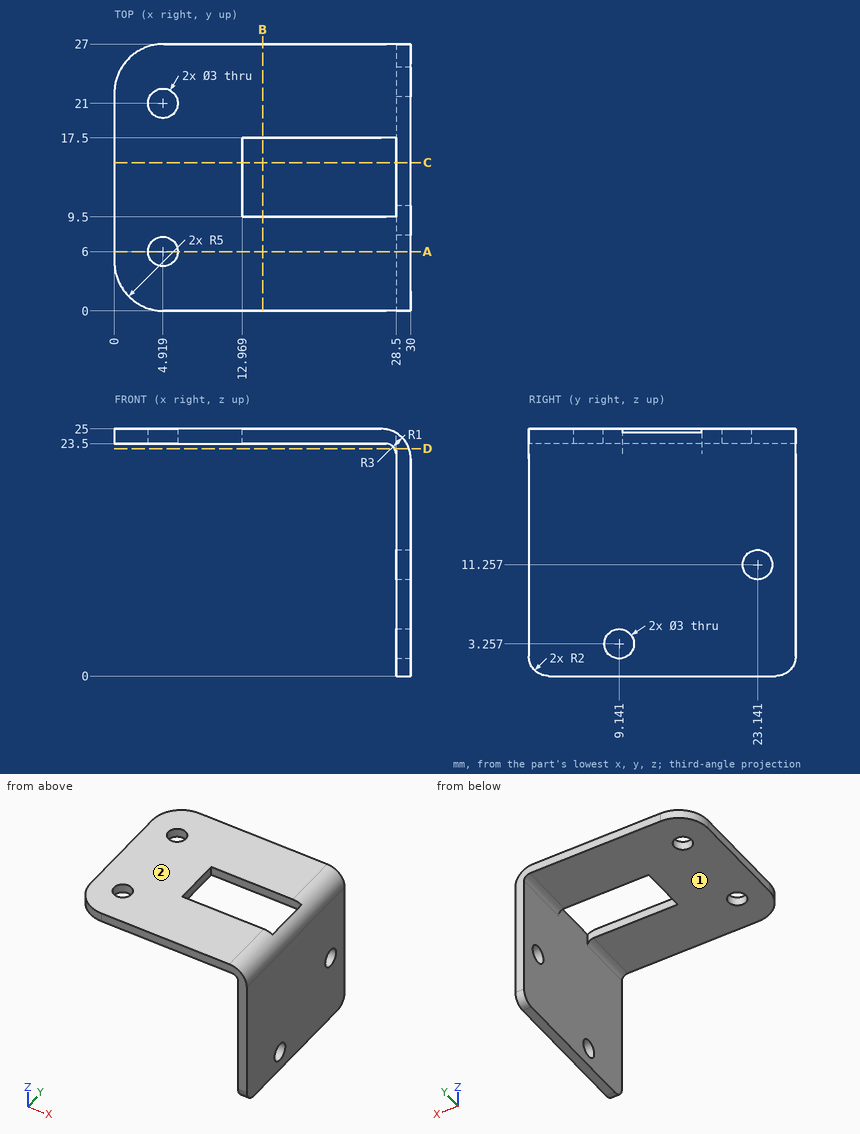
Design review of the part shown in the three views and the two pictorial views. Dimensions are in mm from the part's minimum x, y and z. A direction names the side the tool comes from. Round coordinates to 2 decimals unless told otherwise and drop trailing zeros. Write each loop counter-clockwise with the first axis right and the second up, starting at its lowest first coordinate (ties: lowest second). Pieces come first, ordered by that corner, then holes. Notation, with made-up numbers: (78, -30.5) -> (90, -30.5) arc R21 cw to (90, 2.5) -> close; hole circle Ø4 at (88, -28.5). An arc over 180 degrees is marked (long way). Use one line per item in the form item = value.
1) Take a section at B-B, the plane x = 15. Write out the cut boundary in (y, z), and give its area (3 significant figures).
Found:
outline = (0, 23.5) -> (9.5, 23.5) -> (9.5, 25) -> (0, 25) -> close; (17.5, 23.5) -> (27, 23.5) -> (27, 25) -> (17.5, 25) -> close
area = 28.5 mm2
2) Tool access review of the marked faces 1 and 2: name each direction out of +Z, -Z, +X, -X, +Y, -Y from which nothing blocks a thin tool from reaching the whole face with its end or side.
Found:
face_1 = -Z, -X, +Y, -Y
face_2 = +Z, +X, -X, +Y, -Y
3) Clearance check with flat-ended pins moving along their axes: pin 1 (5 mm diameter, centred on y = 11, z = 11, fed in from -X); pin 2 (8 mm diameter, centred on x = 16, z = 17, fed in from -Y); pin 3 (8 mm diameter, centred on x = 9.5, y = 10, fed in from -Z). State where each tip first meets the part, or that it passes through.
Found:
pin_1 = 28.5
pin_2 = through
pin_3 = 23.5
4) To check wall thickness, follow L1, parallel to Y at x = 22.25, z = 23.75; L2, parallel to X at y = 6.5, z = 20; L3, parallel to Z at x = 17, y = 22.75. State the ranges of each line that lie inside material, in increasing order. Write a range as from..to.
Found:
L1 = 0..9.5, 17.5..27
L2 = 28.5..30
L3 = 23.5..25
5) Take a section at C-C, the plane y = 15. Write out the cut boundary in (x, z).
Found:
outline = (0, 23.5) -> (12.97, 23.5) -> (12.97, 25) -> (0, 25) -> close; (28.5, 0) -> (30, 0) -> (30, 22) arc R3 ccw to (28.5, 24.6) -> close
6) Take a section at A-A, the plane y = 6. Write out the cut boundary in (x, z).
Found:
outline = (0, 23.5) -> (3.42, 23.5) -> (3.42, 25) -> (0, 25) -> close; (6.42, 23.5) -> (27.5, 23.5) arc R1 cw to (28.5, 22.5) -> (28.5, 0) -> (30, 0) -> (30, 22) arc R3 ccw to (27, 25) -> (6.42, 25) -> close
7) Take a section at D-D, the plane z = 23. Write out the cut boundary in (x, y).
Found:
outline = (28.37, 0) -> (29.83, 0) -> (29.83, 27) -> (28.37, 27) -> (28.37, 17.5) -> (28.5, 17.5) -> (28.5, 9.5) -> (28.37, 9.5) -> close
